```python
from build123d import *

# Parameters (mm, degrees)
F0_W     = 13.296557
F0_H     = 13.408921
F0_W_2   = 2.2
F0_H_2   = 2.2
F1_DEPTH = 8


with BuildPart() as f1:
    # F0 (on Right) → F1 (new body)
    with BuildSketch(Plane.YZ):
        with Locations((5.704755, -8.545218)):
            Rectangle(F0_W, F0_H)
        with Locations((0.604655, -13.568869)):
            Rectangle(F0_W_2, F0_H_2, mode=Mode.SUBTRACT)
        with Locations((3.104655, -13.568869)):
            Rectangle(F0_W_2, F0_H_2, mode=Mode.SUBTRACT)
        with Locations((5.604655, -13.568869)):
            Rectangle(F0_W_2, F0_H_2, mode=Mode.SUBTRACT)
        with Locations((0.602163, -11.068871)):
            Rectangle(F0_W_2, F0_H_2, mode=Mode.SUBTRACT)
        with Locations((0.59967, -8.568872)):
            Rectangle(F0_W_2, F0_H_2, mode=Mode.SUBTRACT)
        with Locations((3.102163, -11.068871)):
            Rectangle(F0_W_2, F0_H_2, mode=Mode.SUBTRACT)
        with Locations((5.602163, -11.068871)):
            Rectangle(F0_W_2, F0_H_2, mode=Mode.SUBTRACT)
        with Locations((3.09967, -8.568872)):
            Rectangle(F0_W_2, F0_H_2, mode=Mode.SUBTRACT)
        with Locations((5.59967, -8.568872)):
            Rectangle(F0_W_2, F0_H_2, mode=Mode.SUBTRACT)
        with Locations((8.104655, -13.568869)):
            Rectangle(F0_W_2, F0_H_2, mode=Mode.SUBTRACT)
        with Locations((10.604655, -13.568869)):
            Rectangle(F0_W_2, F0_H_2, mode=Mode.SUBTRACT)
        with Locations((8.102163, -11.068871)):
            Rectangle(F0_W_2, F0_H_2, mode=Mode.SUBTRACT)
        with Locations((8.09967, -8.568872)):
            Rectangle(F0_W_2, F0_H_2, mode=Mode.SUBTRACT)
        with Locations((10.602163, -11.068871)):
            Rectangle(F0_W_2, F0_H_2, mode=Mode.SUBTRACT)
        with Locations((10.59967, -8.568872)):
            Rectangle(F0_W_2, F0_H_2, mode=Mode.SUBTRACT)
        with Locations((0.597177, -6.068873)):
            Rectangle(F0_W_2, F0_H_2, mode=Mode.SUBTRACT)
        with Locations((3.097177, -6.068873)):
            Rectangle(F0_W_2, F0_H_2, mode=Mode.SUBTRACT)
        with Locations((5.597177, -6.068873)):
            Rectangle(F0_W_2, F0_H_2, mode=Mode.SUBTRACT)
        with Locations((0.594684, -3.568874)):
            Rectangle(F0_W_2, F0_H_2, mode=Mode.SUBTRACT)
        with Locations((3.094684, -3.568874)):
            Rectangle(F0_W_2, F0_H_2, mode=Mode.SUBTRACT)
        with Locations((5.594684, -3.568874)):
            Rectangle(F0_W_2, F0_H_2, mode=Mode.SUBTRACT)
        with Locations((8.097177, -6.068873)):
            Rectangle(F0_W_2, F0_H_2, mode=Mode.SUBTRACT)
        with Locations((10.597177, -6.068873)):
            Rectangle(F0_W_2, F0_H_2, mode=Mode.SUBTRACT)
        with Locations((8.094684, -3.568874)):
            Rectangle(F0_W_2, F0_H_2, mode=Mode.SUBTRACT)
        with Locations((10.594684, -3.568874)):
            Rectangle(F0_W_2, F0_H_2, mode=Mode.SUBTRACT)
    extrude(amount=F1_DEPTH)


solid = f1.part
```
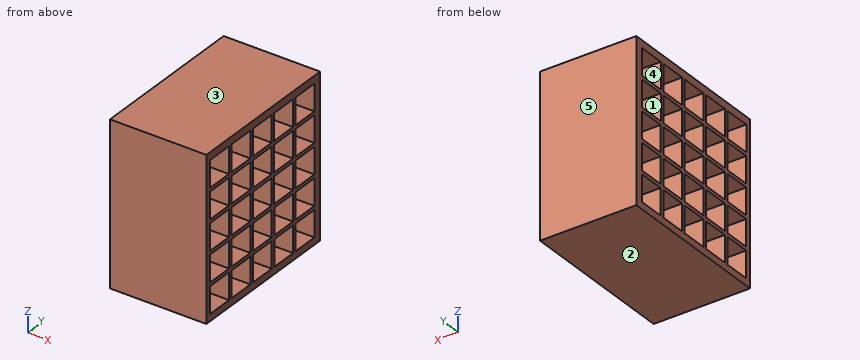
Work out the finished part from the listing and answer in its coordinate system (mm). Face numbers are marked on the shaded views. A direction names the side the tool comes from. Give positions to 0.01 mm unless a question says otherwise; leave off trailing zeros. Write each loop counter-clockwise with the first axis right and the second up, starting at its lowest first coordinate (ties: lowest second). Pieces come first, ordered by that corner, then holes. Notation, with made-up numbers: (-28, 29.5) -> (3, 29.5) arc R11 ccw to (3, 44.5) -> close; hole circle Ø10 at (13.5, 63.25). An arc over 180 degrees is marked (long way). Write each question's results on one line, items separated by ' | '.
1. Find section B-B on y = 3.5. Determine the outline of the cut face in (x, z), and give its area (3 significant figures).
Data:
outline: (0, -15.25) -> (8, -15.25) -> (8, -14.67) -> (0, -14.67) -> close; (0, -12.47) -> (8, -12.47) -> (8, -12.17) -> (0, -12.17) -> close; (0, -9.97) -> (8, -9.97) -> (8, -9.67) -> (0, -9.67) -> close; (0, -7.47) -> (8, -7.47) -> (8, -7.17) -> (0, -7.17) -> close; (0, -4.97) -> (8, -4.97) -> (8, -4.67) -> (0, -4.67) -> close; (0, -2.47) -> (8, -2.47) -> (8, -1.84) -> (0, -1.84) -> close | area: 19.3 mm^2
2. Straight lines are drawn through the part: L1, parallel to Y at x = 6.25, z = -8.75; L2, parallel to Z at x = 6.75, y = 1.5. For each, find the intervals that lie inside material, in ascending order.
Data:
L1: -0.94 to -0.5, 1.7 to 2, 4.2 to 4.5, 6.7 to 7, 9.2 to 9.5, 11.7 to 12.35 | L2: -15.25 to -14.67, -12.47 to -12.17, -9.97 to -9.67, -7.47 to -7.17, -4.97 to -4.67, -2.47 to -1.84
3. Determine the mould class of the marked faces 3, 4 and 5 for opening direction Y: +Y half, -Y half, draft (parallel to the pull), parting line (faces both ways), or undercut.
Data:
face 3: draft | face 4: undercut | face 5: +Y half
4. Find section A-A on z = -9. Determine the outline of the cut face in (x, y).
Data:
outline: (0, -0.94) -> (8, -0.94) -> (8, -0.5) -> (0, -0.5) -> close; (0, 1.7) -> (8, 1.7) -> (8, 2) -> (0, 2) -> close; (0, 4.2) -> (8, 4.2) -> (8, 4.5) -> (0, 4.5) -> close; (0, 6.7) -> (8, 6.7) -> (8, 7) -> (0, 7) -> close; (0, 9.2) -> (8, 9.2) -> (8, 9.5) -> (0, 9.5) -> close; (0, 11.7) -> (8, 11.7) -> (8, 12.35) -> (0, 12.35) -> close
5. Find section C-C on x = 6.75. Give the number of separate pieces and of enclosed holes in the cut face, and give its area (3 significant figures).
Data:
separate pieces: 1 | enclosed holes: 25 | area: 57.3 mm^2
6. A tool of negligible diameter and unlimited length cuts with its end or side. For the marked faces 1 and 2, from which of +Z, -Z, +X, -X, +Y, -Y can it reach the whole face along a straight path? Write none if from no direction.
Data:
face 1: +X, -X | face 2: -Z, +X, -X, +Y, -Y
